Read the model definition and answer for the solid it produces. Units are mm, in the model's axes. Give positions to 0.01 mm unless a question says otherwise; leave off trailing zeros. Order: outer loops, then holes, each group sorted by start corner. A loop starts at its lowest first (then second) coordinate and runs counter-clockwise, first axis right, second up. Notation, with made-up numbers: (-36.5, -8.75) - (7.5, -8.75) arc R36 ccw to (7.5, 26.25) - close; hole circle Ø5 at (-4.75, 39). An arc over 180 degrees is marked (long way). Return JSON: item names as keys, results as strings.
```python
from build123d import *

# Parameters (mm, degrees)
EXTRUDE1_DEPTH = 2.38125
FILLET3_R      = 0.0635


with BuildPart() as part:
    # Sketch1 → Extrude1 (new body)
    with BuildSketch(Plane.XY):
        with BuildLine():
            Line((-6.236773329, -1.1938), (6.236773329, -1.1938))
            ThreePointArc((6.236773329, -1.1938), (0, -6.35), (-6.236773329, -1.1938))
        make_face()
    extrude(amount=EXTRUDE1_DEPTH)

    # Fillet3
    fillet3_edges = [part.edges().sort_by_distance(p)[0] for p in [
        (0, -1.1938, 0),
        (0, -6.35, 0),
        (0, -6.35, 2.38125),
        (-6.236773329, -1.1938, 1.190625),
        (6.236773329, -1.1938, 1.190625),
        (0, -1.1938, 2.38125),
    ]]
    fillet(fillet3_edges, radius=FILLET3_R)


solid = part.part
```
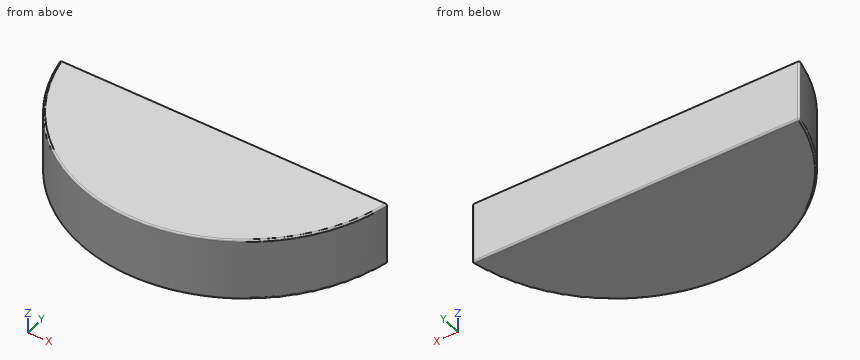
Q1. Consider L1, parallel to Y at x = -1.25, z = 1.9; L2, parallel to X at y = -1.95, z = 0.1; L3, parallel to X at y = -5.7, z = 0.8. Determine where each line is inside the solid, lowest interval first.
Values:
{"L1": "y = -6.23 to -1.19", "L2": "x = -6.04 to 6.04", "L3": "x = -2.8 to 2.8"}
Q2. A cutting plane is placed at A-A (z = 1.05). Write down the section's boundary in (x, y).
Values:
{"outline": "(-6.22, -1.27) arc R6.35 ccw to (6.22, -1.27) arc R0.06 ccw to (6.16, -1.19) - (-6.16, -1.19) arc R0.06 ccw to start"}
Q3. Given pin 1 (1 mm diameter, centred on y = -3.5, z = 0.5, fed in from +X), flat-ended and moving along its own axis, determine where the tip first touches the part or whether it passes through.
Values:
{"pin 1": "stops at x = 5.6"}
